```python
from build123d import *

# Parameters (mm, degrees)
F0_R     = 20
F1_DEPTH = 158
F2_R     = 5
F3_DEPTH = 43
F4_R     = 2


with BuildPart() as f1:
    # F0 (on Right) → F1 (new body)
    with BuildSketch(Plane.YZ):
        Circle(F0_R)
    extrude(amount=F1_DEPTH)

    # F2 (on Top) → F3 (join, symmetric)
    with BuildSketch(Plane.XY):
        with Locations((20, 0)):
            Circle(F2_R)
    extrude(amount=F3_DEPTH, both=True)

    # F4
    f4_edges = [f1.edges().sort_by_distance(p)[0] for p in [
        (158, -20, 0),
    ]]
    fillet(f4_edges, radius=F4_R)


solid = f1.part
```
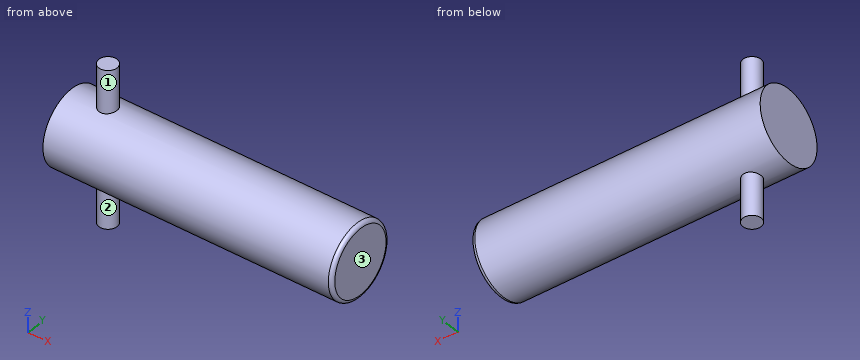
CAD build for the part. Positions are in the model's coordinates, mm. Face numbers are marked on the shaded views. A direction names the side the tool comes from. Round coordinates to 2 decimals unless told otherwise and drop trailing zeros. Write each loop counter-clockwise with the first axis right and the second up, starting at its lowest first coordinate (ties: lowest second). Pieces come first, ordered by that corner, then holes. Notation, with made-up numbers: (-40, 31.5) -> (-34, 31.5) arc R23 ccw to (-34, 65.5) -> close; hole circle Ø7 at (-1, 12). An arc over 180 degrees is marked (long way). Answer in a Markdown table with one row per item. Add a question column.
Item 1: Saw through at B-B, the plane x = 20. Write the cut outline in (y, z).
Item 2: Drop flat-ended pins along their axis: pin 1 Ø12 at (x, z) = (59, -14.5) entering from +Y; pin 2 Ø2 at (x, y) = (65, 8) entering from -Z (3 decimals); pin 3 Ø6 at (x, y) = (126.5, 1.5) entering from +Z; pin 4 Ø10 at (x, z) = (122, -25.5) entering from +Y. Give the stop position or say it passes through.
Item 3: Drill centre lines: line 1 (Z direction, x = 61, y = 5); line 2 (Z direction, x = 69, y = -17.5); line 3 (X direction, y = -3, z = -33.5). Where is each one in solid material? Low to high. Write a range as from..to.
Item 4: Which spindle directions (+Z, -Z, +X, -X, +Y, -Y) get a long thin tool onto all of the face, cutting with end or side? Do the marked faces 1, 2 and 3. Say none if no direction does.
Item 5: Saw through at D-D, the plane x = 119. Write the cut outline in (y, z), then the cut area to 3 significant figures.
Item 6: Saw through at C-C, the plane z = -36.5. Write the cut outline in (x, y).
Item 7: Saw through at A-A, the plane y = 0. Write the cut outline in (x, z), then the cut area to 3 significant figures.
Findings below:
| question | item | result |
|---|---|---|
| 1 | outline | (-5, -43) -> (5, -43) -> (5, -19.36) arc R20 ccw to (5, 19.36) -> (5, 43) -> (-5, 43) -> (-5, 19.36) arc R20 ccw to (-5, -19.36) -> close |
| 2 | pin 1 | stops at y = 18.1 |
| 2 | pin 2 | stops at z = -18.735 |
| 2 | pin 3 | stops at z = 20 |
| 2 | pin 4 | passes through |
| 3 | line 1 | z = -19.36..19.36 |
| 3 | line 2 | z = -9.68..9.68 |
| 3 | line 3 | x = 16..24 |
| 4 | face 1 | +Z |
| 4 | face 2 | -Z |
| 4 | face 3 | +Z, -Z, +X, +Y, -Y |
| 5 | outline | circle Ø40 at (0, 0) |
| 5 | area | 1,260 mm^2 |
| 6 | outline | circle Ø10 at (20, 0) |
| 7 | outline | (0, -20) -> (15, -20) -> (15, -43) -> (25, -43) -> (25, -20) -> (156, -20) arc R2 ccw to (158, -18) -> (158, 18) arc R2 ccw to (156, 20) -> (25, 20) -> (25, 43) -> (15, 43) -> (15, 20) -> (0, 20) -> close |
| 7 | area | 6,780 mm^2 |
